from build123d import *

# Parameters (mm, degrees)
CROQUIS7_R = 5
VACIADO2_T = -1


with BuildPart() as part:
    # Barrer1: sweep along a path in Croquis5
    with BuildLine(Plane(origin=(0, 0, 0), x_dir=(0, 0, -1), z_dir=(1, 0, 0))) as barrer1_path:
        Line((-12, 40), (-12, 82.205417262))
        ThreePointArc((-12, 82.205417262), (-26.544036789, 163.089452311), (-68.354058477, 233.840270104))
        ThreePointArc((-68.354058477, 233.840270104), (-192.782537214, 303.529868669), (-332.920608455, 277.064656453))
        ThreePointArc((-332.920608455, 277.064656453), (-404.710677086, 234.183935346), (-476.226198503, 190.846879685))
    # Croquis7 → Barrer1 (sweep)
    with BuildSketch(Plane(origin=(0, 40, 12), x_dir=(-1, 0, 0), z_dir=(0, 1, 0))):
        Circle(CROQUIS7_R)
    sweep(path=barrer1_path.line)

    # Vaciado2
    vaciado2_openings = [part.faces().sort_by_distance(p)[0] for p in [
        (0, 190.846879685, 476.226198503),
        (0, 40, 12),
    ]]
    offset(amount=VACIADO2_T, openings=vaciado2_openings, kind=Kind.INTERSECTION)


solid = part.part
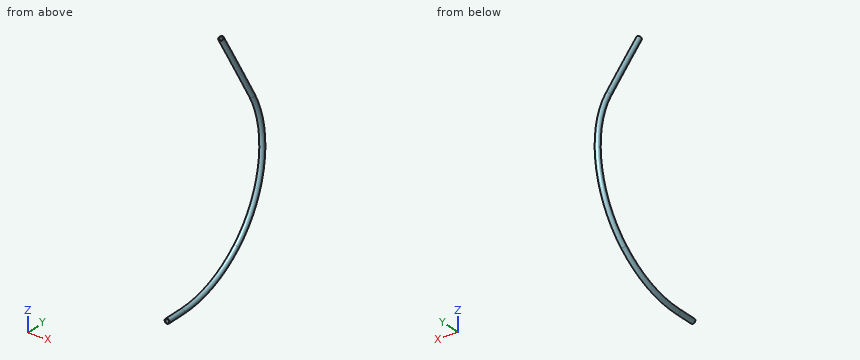
Verification items for the finished model (mm, model axes). Round coordinates to 2 decimals unless told otherwise and drop trailing zeros. Write each loop counter-clockwise with the first axis right and the second up, starting at its lowest first coordinate (ties: lowest second). Pieces come first, ordered by that corner, then holes.
(1) Material ranges on line 1 (Z direction, x = 0, y = 49); line 2 (Z direction, x = -3.5, y = 60); line 3 (Y direction, x = 1.75, z = 342), recorded low to high.
Returned:
line 1: z = 7 to 8, 16 to 17
line 2: z = 8.43 to 10.06, 13.94 to 15.57
line 3: y = 266.23 to 267.49, 275.86 to 277.12
(2) Section check A-A (x = 0). Enter the section's corners in (y, z), plus the area to 3 significant figures.
Returned:
outline: (40, 7) - (82.21, 7) arc R237.18 ccw to (237.11, 64.57) arc R213.76 ccw to (281.37, 335.47) arc R13135.17 ccw to (195.11, 478.83) - (194.26, 478.31) arc R13134.17 cw to (280.51, 334.96) arc R212.76 cw to (236.45, 65.32) arc R236.18 cw to (82.21, 8) - (40, 8) - close; (40, 16) - (82.21, 16) arc R228.18 ccw to (231.23, 71.38) arc R204.76 ccw to (273.62, 330.88) arc R13126.17 ccw to (187.43, 474.14) - (186.58, 473.62) arc R13125.17 cw to (272.76, 330.37) arc R203.76 cw to (230.57, 72.14) arc R227.18 cw to (82.21, 17) - (40, 17) - close
area: 1,330 mm2
(3) Section check B-B (y = 261.5). Give the number of separate pieces and of enclosed holes in the cut face, plus the area to 3 significant figures.
Returned:
separate pieces: 2
enclosed holes: 2
area: 101 mm2
(4) Depth check by flat-ended pin: pin 1 Ø1.5 at (x, z) = (1, 242) entering from -Y; pin 2 Ø4 at (x, z) = (-1, 250) entering from +Y; pin 3 Ø5 at (x, y) = (1.5, 186.5) entering from -Z. Enter the tip coordinate at first touch or a pass-through.
Returned:
pin 1: stops at y = 300.65
pin 2: stops at y = 310.15
pin 3: stops at z = 30.07
